For this review, take the finished solid that the model builds, in its own axes (mm). Face numbers are marked on the shaded views. A direction names the side the tool comes from. Round coordinates to 2 decimals unless told otherwise and drop trailing zeros. Write each loop counter-clockwise with the first axis right and the second up, starting at its lowest first coordinate (ties: lowest second). Pieces come first, ordered by that corner, then holes. Notation, with made-up numbers: M -22,27 L 33,27 A21 cw 33,40 Z; hole C 1,35 d1. An arc over 180 degrees is marked long. Answer in a Markdown table with one row per item.
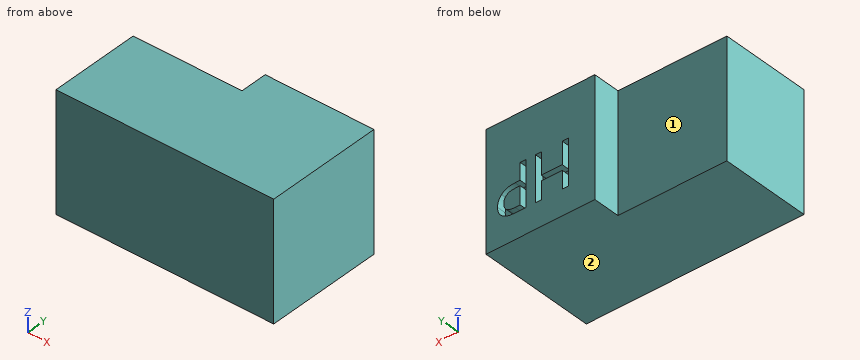
Autodesk Inventor part; units mm, degrees
ref_plane "YZ Plane" through (0, 0, 0) normal (1, 0, 0) x (0, 1, 0)
ref_plane "XZ Plane" through (0, 0, 0) normal (0, 1, 0) x (-1, 0, 0)
ref_plane "XY Plane" through (0, 0, 0) normal (0, 0, 1) x (1, 0, 0)
sketch "Sketch1" plane through (0, 0, 0) normal (0, 1, 0) x (-1, 0, 0)
  line L0 (-120, -65) -> (120, -65)
  line L1 (120, -65) -> (120, 65)
  line L2 (120, 65) -> (-120, 65)
  line L3 (-120, 65) -> (-120, -65)
  line L4 (-120, -65) -> (120, 65) construction
  line L5 (120, -65) -> (-120, 65) construction
  line L6 (0, 65) -> (0, -65)
  point P0 (0, 0)
  dimension "d0" = 240
  dimension "d1" = 130
  dimension "d4" = 120
extrude "Extrusion1" add sketch "Sketch1" along normal blind 100
extrude "Extrusion2" add sketch "Sketch1" along normal blind 30 from surface at 100 contours L3 L2 L6 L0
sketch "Sketch2" plane through (0, 130, -65) normal (0, 1, 0) x (1, 0, 0)
  line L0 (24.228, -27.798) -> (40.6948, -27.798) construction
  line L1 (40.6948, -27.798) -> (40.6948, -38.1545) construction
  line L2 (40.6948, -38.1545) -> (24.228, -38.1545) construction
  line L3 (24.228, -38.1545) -> (24.228, -27.798) construction
  line L4 (65.5975, -77.798) -> (58.9525, -77.798)
  line L5 (58.9525, -77.798) -> (58.9525, -53.3247)
  line L6 (58.9525, -53.3247) -> (35.9379, -53.3247)
  line L7 (35.9379, -53.3247) -> (35.9379, -77.798)
  line L8 (35.9379, -77.798) -> (29.2928, -77.798)
  line L9 (29.2928, -77.798) -> (29.2928, -27.798)
  line L10 (29.2928, -27.798) -> (35.9379, -27.798)
  line L11 (35.9379, -27.798) -> (35.9379, -47.409)
  line L12 (35.9379, -47.409) -> (58.9525, -47.409)
  line L13 (58.9525, -47.409) -> (58.9525, -27.798)
  line L14 (58.9525, -27.798) -> (65.5975, -27.798)
  line L15 (65.5975, -27.798) -> (65.5975, -77.798)
  spline S0 degree 2 poles (107.3317, -42.8709) (107.3317, -46.1124) (105.0222, -51.9471) (102.9557, -53.973) knots 0 0 0 1 2 2 2
  spline S1 degree 2 poles (102.9557, -53.973) (100.3625, -56.5257) (93.3528, -59.1594) (88.0043, -59.1594) knots 0 0 0 1 2 2 2
  line L16 (88.0043, -59.1594) -> (82.3723, -59.1594)
  line L17 (82.3723, -59.1594) -> (82.3723, -77.798)
  line L18 (82.3723, -77.798) -> (75.7272, -77.798)
  line L19 (75.7272, -77.798) -> (75.7272, -27.798)
  line L20 (75.7272, -27.798) -> (88.288, -27.798)
  spline S2 degree 2 poles (88.288, -27.798) (92.745, -27.798) (98.9849, -29.2566) (101.3755, -30.9179) knots 0 0 0 1 2 2 2
  spline S3 degree 2 poles (101.3755, -30.9179) (104.1713, -32.8223) (107.3317, -38.6975) (107.3317, -42.8709) knots 0 0 0 1 2 2 2
  spline S4 degree 2 poles (100.403, -43.0735) (100.403, -40.4803) (98.6202, -36.6715) (96.7969, -35.456) knots 0 0 0 1 2 2 2
  spline S5 degree 2 poles (96.7969, -35.456) (95.2167, -34.4025) (91.0027, -33.5516) (87.8828, -33.5516) knots 0 0 0 1 2 2 2
  line L21 (87.8828, -33.5516) -> (82.3723, -33.5516)
  line L22 (82.3723, -33.5516) -> (82.3723, -53.4868)
  line L23 (82.3723, -53.4868) -> (86.9103, -53.4868)
  spline S6 degree 2 poles (86.9103, -53.4868) (90.9622, -53.4868) (95.946, -52.1902) (97.5667, -50.4884) knots 0 0 0 1 2 2 2
  spline S7 degree 2 poles (97.5667, -50.4884) (99.0659, -48.9892) (100.403, -45.4641) (100.403, -43.0735) knots 0 0 0 1 2 2 2
  point P0 (0, -65)
  point P1 (67.1766, -110.0367)
extrude "Extrusion3" cut sketch "Sketch2" against normal blind 10
properties part number "HotPlate"
Q1. Take a section at C-C (y = 108). State the section outline as (x, z) points, then the cut area to 3 significant figures.
Found:
| item | result |
|---|---|
| outline | M 0,-65 L 120,-65 L 120,65 L 0,65 Z |
| area | 15,600 mm² |
Q2. For probe 1 along Z at (x, y) = (47, 122); probe 2 along Y at (x, z) = (-100.5, -6); probe 3 along X at (y, z) = (116, 49), list the stretches that pass through material, from the lowest coordinate up.
Found:
| item | result |
|---|---|
| probe 1 | -65 to -17.59, -11.68 to 65 |
| probe 2 | 0 to 100 |
| probe 3 | 0 to 120 |
Q3. Machinability: for the marked faces 1 and 2, which of the approach directions +Z, -Z, +X, -X, +Y, -Y give a long, thin tool a straight path to every point of the face, cutting with its end or side? Answer none if there is none.
Found:
| item | result |
|---|---|
| face 1 | +Z, -Z, -X, +Y |
| face 2 | -Z, +X, -X, +Y, -Y |
Q4. Take a section at D-D (x = -47). State the section outline as (y, z) points.
Found:
| item | result |
|---|---|
| outline | M 0,-65 L 100,-65 L 100,65 L 0,65 Z |
Q5. Insertion check: P1, Ø9, axis at y = 108, z = 24.5, coming from the -X side; P2, Ø1.5, axis at x = -87.5, z = -21.5, coming from the -Y side; P3, Ø2, axis at x = -14.5, z = -5, coming from the +Y side. Each pin has a flat end and moves straight along its axis. Give the tip position at first contact, or say it passes through.
Found:
| item | result |
|---|---|
| P1 | x = 0 |
| P2 | y = 0 |
| P3 | y = 100 |
Q6. Take a section at B-B (z = 45). State the section outline as (x, y) points, then the cut area to 3 significant figures.
Found:
| item | result |
|---|---|
| outline | M -120,0 L 120,0 L 120,130 L 0,130 L 0,100 L -120,100 Z |
| area | 27,600 mm² |
Q7. Take a section at A-A (x = 63). State the section outline as (y, z) points.
Found:
| item | result |
|---|---|
| outline | M 0,-65 L 130,-65 L 130,-37.2 L 120,-37.2 L 120,12.8 L 130,12.8 L 130,65 L 0,65 Z |
